```python
from build123d import *

# Parameters (mm, degrees)
F1_DEPTH = 37.0078
F2_W     = 24.9682
F2_H     = 8.9916
F3_DEPTH = 24.9428
F4_W     = 16.9418
F4_H     = 20.8534
F5_DEPTH = 24.003


with BuildPart() as f1:
    # F0 (on Front) → F1 (new body)
    with BuildSketch(Plane.XZ):
        Polygon((0, 35.9918), (0, 0), (56.007, 0), (56.007, 35.9918), (40.005, 35.9918), (40.005, 24.384), (16.002, 24.384), (16.002, 35.9918), align=None)
    extrude(amount=F1_DEPTH)

    # F2 (on face) → F3 (cut)
    with BuildSketch(Plane.XZ.offset(37.0078)):
        with Locations((12.4841, 4.4958)):
            Rectangle(F2_W, F2_H)
    extrude(amount=-F3_DEPTH, mode=Mode.SUBTRACT)

    # F4 (on face) → F5 (cut)
    with BuildSketch(Plane.YZ.offset(56.007)):
        with Locations((-8.4709, 10.4267)):
            Rectangle(F4_W, F4_H)
    extrude(amount=-F5_DEPTH, mode=Mode.SUBTRACT)


solid = f1.part
```
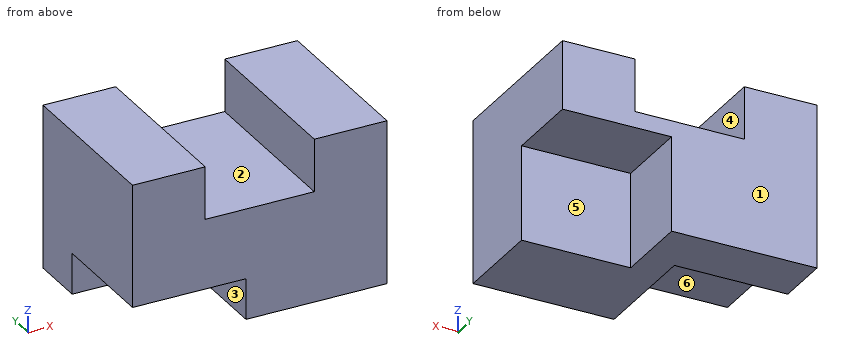
Here's how the part is built. I have some questions about the finished solid (model axes, mm). Face numbers are marked on the shaded views. A direction names the side the tool comes from. Give positions to 0.01 mm unless a question says otherwise; leave off trailing zeros. Loops run counter-clockwise (first coordinate to the right, second up) from the corner with the lowest first, then second, coordinate; pieces in that order, holes last. Notation, with made-up numbers: (37, 40.5) -> (92, 40.5) arc R28 ccw to (92, 70.5) -> close; hole circle Ø11 at (55, 80.5). An arc over 180 degrees is marked (long way). Use one line per item in the form item = value. Start each with the question number.
1) Please list where these lines run through material, in increasing order: line 1 along X through (y, z) = (-32.5, 33.5) (3 decimals); line 2 along Z through (x, y) = (47.5, -5); line 3 along Z through (x, y) = (34.5, -5).
2) Imagine slicing it at D-D (x = 44.5). Please give me the cut outline in (y, z), then the cut area to 3 significant figures.
3) Imagine slicing it at A-A (y = -13.5). Please give me the cut outline in (x, z) (3 decimals), then the cut area to 3 significant figures.
4) Imagine slicing it at C-C (z = 4.5). Please give me the cut outline in (x, y) (3 decimals).
5) Which directions (+Z, -Z, +X, -X, +Y, -Y) give clear straight access to the entire face, cutting with the end or side of a thin tool? Please do the marked faces 4, 5 and 6.
6) Imagine slicing it at B-B (z = 28). Please give me the cut outline in (x, y) (3 decimals), then the cut area to 3 significant figures.
7) Thinking about a two-plate mould opening in X: for the marked faces 1, 2 and 3, which applies, +X half, -X half, draft (parallel to the pull), parting line (faces both ways), or undercut?
8) For P1, Ø19, axis at x = 26, y = -19.5, coming from the +Z side; P2, Ø5, axis at y = -12.5, z = 7, coming from the +X side; P3, Ø10.5, axis at x = 47, z = 15.5, coming from the +Y side, each with a flat end and sliding along its axis, tell me the tip position at first contact or that it passes through.
Check values:
q1.line_1 = 0 to 16.002, 40.005 to 56.007
q1.line_2 = 20.85 to 35.99
q1.line_3 = 20.85 to 24.38
q2.outline = (-37.01, 0) -> (-16.94, 0) -> (-16.94, 20.85) -> (0, 20.85) -> (0, 35.99) -> (-37.01, 35.99) -> close
q2.area = 979 mm^2
q3.outline = (0, 8.992) -> (24.968, 8.992) -> (24.968, 0) -> (32.004, 0) -> (32.004, 20.853) -> (56.007, 20.853) -> (56.007, 35.992) -> (40.005, 35.992) -> (40.005, 24.384) -> (16.002, 24.384) -> (16.002, 35.992) -> (0, 35.992) -> close
q3.area = 1,010 mm^2
q4.outline = (0, -12.065) -> (24.968, -12.065) -> (24.968, -37.008) -> (56.007, -37.008) -> (56.007, -16.942) -> (32.004, -16.942) -> (32.004, 0) -> (0, 0) -> close
q5.face_4 = +Z, +Y, -Y
q5.face_5 = -Z, +X, +Y
q5.face_6 = -Z, -X, -Y
q6.outline = (0, -37.008) -> (16.002, -37.008) -> (16.002, 0) -> (0, 0) -> close; (40.005, -37.008) -> (56.007, -37.008) -> (56.007, 0) -> (40.005, 0) -> close
q6.area = 1,180 mm^2
q7.face_1 = draft
q7.face_2 = undercut
q7.face_3 = -X half
q8.P1 = 24.38
q8.P2 = 32
q8.P3 = -16.94
